Design review of the part built by this model. Coordinates are the model's own, in mm. Coordinates: 2 decimals unless noted, no trailing zeros. Loops run counter-clockwise (first coordinate to the right, second up) from the corner with the lowest first, then second, coordinate; pieces in that order, holes last. Notation, with made-up numbers: (75, 77.5) -> (81, 77.5) arc R8 ccw to (81, 87.5) -> close; hole circle Ø9 at (71, 4). An arc over 180 degrees is marked (long way). Use a Markdown table: item, result. Add a question column.
Q1. Take a section at C-C on y = 8. Write out the cut boundary in (x, z), plus the area to 3 significant figures.
Q2. Draft analysis for pull direction X (two halves, no side actions). For faces 1 (the face through (4, -4, 7)), 2 (the face through (-0.65, 9.01, 3.45)), 3 (the face through (-4.336, -19.524, 3.451)), state which applies: pulls with the +X half, pulls with the -X half, needs draft (parallel to the pull), parting line crosses it, or undercut.
Q3. For probe 1 along Y at (x, z) = (0, 5.5); probe 2 along Y at (x, z) = (-8, 5); probe 3 along X at (y, z) = (2, 2.75), list the stretches that pass through material, from the lowest coordinate up.
Q4. Take a section at A-A on x = 0. Write out the cut boundary in (y, z), plus the area to 3 significant figures.
Q5. Take a section at B-B on z = 5.5. Write out the cut boundary in (x, y), plus the area to 3 significant figures.
Q6. Clearance check with flat-ended pins moving along their axes: pin 1 Ø2 at (y, z) = (-2.5, 4) entering from +X; pin 2 Ø2 at (y, z) = (-13, 3) entering from +X; pin 3 Ø4 at (y, z) = (5, 6) entering from -X. State where each tip first meets the part, or that it passes through.
from build123d import *

# Parameters (mm, degrees)
ESQUISSE1_R        = 20
ESQUISSE1_R_2      = 5
BOSS_EXTRU_1_DEPTH = 7
D_GAGEMENT_M21_D   = 2.4


with BuildPart() as part:
    # Esquisse1 → Boss.-Extru.1 (new body)
    with BuildSketch(Plane.XY):
        Circle(ESQUISSE1_R)
        Circle(ESQUISSE1_R_2, mode=Mode.SUBTRACT)
    extrude(amount=BOSS_EXTRU_1_DEPTH)

    # Dégagement M21 (through all)
    with Locations(Plane.XY.offset(7)):
        with Locations((0, 8), (8, 0), (0, -8), (-8, 0), (0, 0)):
            Hole(D_GAGEMENT_M21_D / 2)


solid = part.part
Answer list:
| question | item | result |
|---|---|---|
| 1 | outline | (-18.33, 0) -> (-1.2, 0) -> (-1.2, 7) -> (-18.33, 7) -> close; (1.2, 0) -> (18.33, 0) -> (18.33, 7) -> (1.2, 7) -> close |
| 1 | area | 240 mm² |
| 2 | face 1 | needs draft |
| 2 | face 2 | undercut |
| 2 | face 3 | parting line crosses it |
| 3 | probe 1 | -20 to -9.2, -6.8 to -5, 5 to 6.8, 9.2 to 20 |
| 3 | probe 2 | -18.33 to -1.2, 1.2 to 18.33 |
| 3 | probe 3 | -19.9 to -4.58, 4.58 to 19.9 |
| 4 | outline | (-20, 0) -> (-9.2, 0) -> (-9.2, 7) -> (-20, 7) -> close; (-6.8, 0) -> (-5, 0) -> (-5, 7) -> (-6.8, 7) -> close; (5, 0) -> (6.8, 0) -> (6.8, 7) -> (5, 7) -> close; (9.2, 0) -> (20, 0) -> (20, 7) -> (9.2, 7) -> close |
| 4 | area | 176 mm² |
| 5 | outline | circle Ø40 at (0, 0); hole circle Ø2.4 at (-8, 0); hole circle Ø10 at (0, 0); hole circle Ø2.4 at (0, -8); hole circle Ø2.4 at (0, 8); hole circle Ø2.4 at (8, 0) |
| 5 | area | 1,160 mm² |
| 6 | pin 1 | x = 19.94 |
| 6 | pin 2 | x = 16 |
| 6 | pin 3 | x = -19.77 |
